Verification items for the finished model (mm, model axes). A direction names the side the tool comes from. Round coordinates to 2 decimals unless told otherwise and drop trailing zeros. Loops run counter-clockwise (first coordinate to the right, second up) from the corner with the lowest first, then second, coordinate; pieces in that order, holes last. Notation, with made-up numbers: (19, 49) - (61, 49) arc R22 cw to (61, 69) - close; hole circle Ø3 at (24.5, -11.75). An arc over 180 degrees is marked (long way). Use a Markdown table: item, result. Add a question column.
```python
from build123d import *

# Parameters (mm, degrees)
SKETCH1_W           = 45.323908176
SKETCH1_H           = 26.783449256
SKETCH1_R           = 4.05
SKETCH1_R_2         = 4.1
SKETCH1_R_3         = 4.2
SKETCH1_R_4         = 6.05
SKETCH1_R_5         = 6.1
SKETCH1_R_6         = 6.2
BOSS_EXTRUDE1_DEPTH = 15
CUT_EXTRUDE1_DEPTH  = 1


with BuildPart() as part:
    # Sketch1 → Boss-Extrude1 (new body)
    with BuildSketch(Plane(origin=(0, 0, 0), x_dir=(1, 0, 0), z_dir=(0, 1, 0))):
        Rectangle(SKETCH1_W, SKETCH1_H)
        with Locations(Location((-14.194850363, -5.790004753, 0), (0, 0, 270))):
            Circle(SKETCH1_R, mode=Mode.SUBTRACT)
        with Locations(Location((0.622581156, -5.914520985, 0), (0, 0, 270))):
            Circle(SKETCH1_R_2, mode=Mode.SUBTRACT)
        with Locations(Location((15.190980213, -6.288069678, 0), (0, 0, 270))):
            Circle(SKETCH1_R_3, mode=Mode.SUBTRACT)
        with Locations(Location((-14.443882825, 5.790004753, 0), (0, 0, 270))):
            Circle(SKETCH1_R_4, mode=Mode.SUBTRACT)
        with Locations(Location((0.124516231, 5.790004753, 0), (0, 0, 270))):
            Circle(SKETCH1_R_5, mode=Mode.SUBTRACT)
        with Locations(Location((14.94194775, 5.665488522, 0), (0, 0, 270))):
            Circle(SKETCH1_R_6, mode=Mode.SUBTRACT)
    extrude(amount=BOSS_EXTRUDE1_DEPTH)

    # Sketch2 → Cut-Extrude1 (cut)
    with BuildSketch(Plane(origin=(0, 15, 0), x_dir=(1, 0, 0), z_dir=(0, 1, 0))):
        Polygon((-6.12211696, 0), (-6.12211696, -0.70072423), (-8.851253436, -0.70072423), (-8.851253436, -1.80713091), (-6.12211696, -1.80713091), (-6.12211696, -2.839777144), (-4.536267386, -1.25392757), align=None)
    extrude(amount=-CUT_EXTRUDE1_DEPTH, mode=Mode.SUBTRACT)


solid = part.part
```
Q1. Section check D-D on x = 14. Record the cut outline in (y, z).
Q2. Release check for a two-part mould opening along X. For faces 3 (the face through (-22.662, 7, 0)), 4 (the face through (19.355, 7.395, 5.741)), 5 (the face through (0, 7, 13.392)) record: +X half, -X half, draft (parallel to the pull), parting line (faces both ways), or undercut.
Q3. Section check B-B on z = -7. Record the cut outline in (x, y), plus the area to 3 significant figures.
Q4. Section check C-C on y = 3.5. Record the cut outline in (x, z).
Q5. Thickness scan on line 1 along Z through (x, y) = (15.5, 6.75); line 2 along X through (y, z) = (10.5, -1); line 3 along Z through (x, y) = (18.5, 12.5). Record the ranges inside material, lowest first.
Q6. Section check A-A on x = -16. Record the cut outline in (y, z), plus the area to 3 significant figures.
Q7. Set-up check for faces 1 (the face through (-8.851, 14.5, 1.2)), 2 (the face through (-5, 0, 0)): record each of +Z, -Z, +X, -X, +Y, -Y from which the full face is reachable in a straight line by a thin tool's end or side.
Determined:
| question | item | result |
|---|---|---|
| 1 | outline | (0, -13.39) - (15, -13.39) - (15, -11.79) - (0, -11.79) - close; (0, 0.46) - (15, 0.46) - (15, 2.26) - (0, 2.26) - close; (0, 10.32) - (15, 10.32) - (15, 13.39) - (0, 13.39) - close |
| 2 | face 3 | -X half |
| 2 | face 4 | undercut |
| 2 | face 5 | draft |
| 3 | outline | (-22.66, 0) - (-20.37, 0) - (-20.37, 15) - (-22.66, 15) - close; (-8.52, 0) - (-5.85, 0) - (-5.85, 15) - (-8.52, 15) - close; (6.1, 0) - (8.89, 0) - (8.89, 15) - (6.1, 15) - close; (21, 0) - (22.66, 0) - (22.66, 15) - (21, 15) - close |
| 3 | area | 141 mm² |
| 4 | outline | (-22.66, -13.39) - (22.66, -13.39) - (22.66, 13.39) - (-22.66, 13.39) - close; hole circle Ø12.1 at (-14.44, -5.79); hole circle Ø8.1 at (-14.19, 5.79); hole circle Ø12.2 at (0.12, -5.79); hole circle Ø8.2 at (0.62, 5.91); hole circle Ø12.4 at (14.94, -5.67); hole circle Ø8.4 at (15.19, 6.29) |
| 5 | line 1 | z = -13.39 to -11.84, 0.51 to 2.1, 10.48 to 13.39 |
| 5 | line 2 | x = -22.66 to -18.14, -10.75 to -3.65, 3.9 to 10.86, 19.03 to 22.66 |
| 5 | line 3 | z = -13.39 to -10.74, -0.59 to 3.7, 8.87 to 13.39 |
| 6 | outline | (0, -13.39) - (15, -13.39) - (15, -11.64) - (0, -11.64) - close; (0, 0.06) - (15, 0.06) - (15, 2.16) - (0, 2.16) - close; (0, 9.42) - (15, 9.42) - (15, 13.39) - (0, 13.39) - close |
| 6 | area | 118 mm² |
| 7 | face 1 | +Y |
| 7 | face 2 | +Z, -Z, +X, -X, -Y |
